from build123d import *

# Parameters (mm, degrees)
SKETCH1_R           = 2
BOSS_EXTRUDE1_DEPTH = 6


with BuildPart() as part:
    # Sketch1 → Boss-Extrude1 (new body)
    with BuildSketch(Plane.XY):
        with BuildLine():
            Line((-3.5, 0), (-3.5, 28))
            ThreePointArc((-3.5, 28), (0, 31.5), (3.5, 28))
            Line((3.5, 28), (3.5, 0))
            ThreePointArc((3.5, 0), (0, -3.5), (-3.5, 0))
        make_face()
        Circle(SKETCH1_R, mode=Mode.SUBTRACT)
        with Locations((0, 7)):
            Circle(SKETCH1_R, mode=Mode.SUBTRACT)
        with Locations((0, 14)):
            Circle(SKETCH1_R, mode=Mode.SUBTRACT)
        with Locations((0, 21)):
            Circle(SKETCH1_R, mode=Mode.SUBTRACT)
        with Locations((0, 28)):
            Circle(SKETCH1_R, mode=Mode.SUBTRACT)
    extrude(amount=BOSS_EXTRUDE1_DEPTH)


solid = part.part
Read the model definition and answer for the solid it produces. Units are mm, in the model's axes. Round coordinates to 2 decimals unless told otherwise and drop trailing zeros. Loops run counter-clockwise (first coordinate to the right, second up) from the corner with the lowest first, then second, coordinate; pieces in that order, holes last.
Q1. Section B-B on x = 0 is taken. Write down the section's boundary in (y, z), and give its area (3 significant figures).
Q2. Section D-D on x = 1.5 is taken. Write down the section's boundary in (y, z), and give its area (3 significant figures).
Q3. This flat-tipped pin is pushed along its axis until it touches: pin 1 (3 mm diameter, centred on x = -1.5, z = 1, fed in from +Y). Where does it stop, or does it pass through?
Q4. Consider probe 1 along Y at (x, z) = (0, 3.1); probe 2 along Y at (x, z) = (0.5, 4.6); probe 3 along X at (y, z) = (22, 3.45). Determine where each line is inside the solid, lowest interval first.
Q5. Section A-A on y = 14 is taken. Write down the section's boundary in (x, z).
Q6. Determine the mould class of faces 1 (the face through (2.4, 14.2, 0)), 2 (the face through (0, 26, 3)), 3 (the face through (-0.1, 31.5, 3)) for opening direction X: released by +X, released by -X, zero draft, split by the parting line, or undercut.
Q7. Section C-C on z = 2.25 is taken. Write down the section's boundary in (x, y), and give its area (3 significant figures).
Output:
1. outline: (-3.5, 0) - (-2, 0) - (-2, 6) - (-3.5, 6) - close; (2, 0) - (5, 0) - (5, 6) - (2, 6) - close; (9, 0) - (12, 0) - (12, 6) - (9, 6) - close; (16, 0) - (19, 0) - (19, 6) - (16, 6) - close; (23, 0) - (26, 0) - (26, 6) - (23, 6) - close; (30, 0) - (31.5, 0) - (31.5, 6) - (30, 6) - close
1. area: 90.0 mm2
2. outline: (-3.16, 0) - (-1.32, 0) - (-1.32, 6) - (-3.16, 6) - close; (1.32, 0) - (5.68, 0) - (5.68, 6) - (1.32, 6) - close; (8.32, 0) - (12.68, 0) - (12.68, 6) - (8.32, 6) - close; (15.32, 0) - (19.68, 0) - (19.68, 6) - (15.32, 6) - close; (22.32, 0) - (26.68, 0) - (26.68, 6) - (22.32, 6) - close; (29.32, 0) - (31.16, 0) - (31.16, 6) - (29.32, 6) - close
2. area: 127 mm2
3. pin 1: stops at y = 31.5
4. probe 1: y = -3.5 to -2, 2 to 5, 9 to 12, 16 to 19, 23 to 26, 30 to 31.5
4. probe 2: y = -3.46 to -1.94, 1.94 to 5.06, 8.94 to 12.06, 15.94 to 19.06, 22.94 to 26.06, 29.94 to 31.46
4. probe 3: x = -3.5 to -1.73, 1.73 to 3.5
5. outline: (-3.5, 0) - (-2, 0) - (-2, 6) - (-3.5, 6) - close; (2, 0) - (3.5, 0) - (3.5, 6) - (2, 6) - close
6. face 1: zero draft
6. face 2: undercut
6. face 3: split by the parting line
7. outline: (-3.5, 0) arc R3.5 ccw to (3.5, 0) - (3.5, 28) arc R3.5 ccw to (-3.5, 28) - close; hole circle Ø4 at (0, 0); hole circle Ø4 at (0, 7); hole circle Ø4 at (0, 14); hole circle Ø4 at (0, 21); hole circle Ø4 at (0, 28)
7. area: 172 mm2
